from build123d import *

# Parameters (mm, degrees)
F0_W     = 25.4
F0_H     = 25.4
F1_DEPTH = 50.8
F2_R     = 5.08
F3_R     = 5.08


with BuildPart() as f1:
    # F0 (on Top) → F1 (new body)
    with BuildSketch(Plane.XY):
        with Locations((-35.092446, -26.748407)):
            Rectangle(F0_W, F0_H)
    extrude(amount=F1_DEPTH)

    # F2
    f2_edges = [f1.edges().sort_by_distance(p)[0] for p in [
        (-47.792446, -26.748407, 50.8),
    ]]
    fillet(f2_edges, radius=F2_R)

    # F3
    f3_edges = [f1.edges().sort_by_distance(p)[0] for p in [
        (-32.552446, -39.448407, 50.8),
        (-22.392446, -26.748407, 50.8),
        (-32.552446, -14.048407, 50.8),
    ]]
    fillet(f3_edges, radius=F3_R)


solid = f1.part
For this review, take the finished solid that the model builds, in its own axes (mm). Round coordinates to 2 decimals unless told otherwise and drop trailing zeros. Loops run counter-clockwise (first coordinate to the right, second up) from the corner with the lowest first, then second, coordinate; pieces in that order, holes last. Notation, with made-up numbers: (20, 25) - (58, 25) arc R17 ccw to (58, 57) - close; hole circle Ø7 at (75, 49.25). An arc over 180 degrees is marked (long way). Use one line per item in the form item = value.
1) Wall thickness on probe 1 along Z at (x, y) = (-40.75, -34.5); probe 2 along Z at (x, y) = (-31, -36.5); probe 3 along X at (y, z) = (-33.75, 48.5): over which ranges is each line inside the solid? List them lowest first.
Solutions:
probe_1 = 0 to 50.8
probe_2 = 0 to 50.33
probe_3 = -46.96 to -23.22
2) We need section A-A on z = 32.5. Write out the cut boundary in (x, y), then the cut area to 3 significant figures.
Solutions:
outline = (-47.79, -34.37) arc R5.08 ccw to (-42.71, -39.45) - (-22.39, -39.45) - (-22.39, -14.05) - (-42.71, -14.05) arc R5.08 ccw to (-47.79, -19.13) - close
area = 634 mm2
3) We need section B-B on x = -24. Write out the cut boundary in (y, z), then the cut area to 3 significant figures.
Solutions:
outline = (-39.45, 0) - (-14.05, 0) - (-14.05, 45.72) arc R5.08 ccw to (-15.66, 49.43) - (-37.84, 49.43) arc R5.08 ccw to (-39.45, 45.72) - close
area = 1,250 mm2
